Work out the finished part from the listing and answer in its coordinate system (mm). A direction names the side the tool comes from. Coordinates: 2 decimals unless noted, no trailing zeros. Order: outer loops, then holes, each group sorted by start corner. A loop starts at its lowest first (then second) coordinate and runs counter-clockwise, first axis right, second up. Notation, with made-up numbers: M -14,41.5 L -3,41.5 A26 cw -3,57.5 Z; hole C -16.75,-3.75 d3. An arc over 180 degrees is marked long. Use a Markdown table: item, result.
from build123d import *

# Parameters (mm, degrees)
SKETCH_1_R               = 1.65
SKETCH_1_W               = 14
SKETCH_1_H               = 4
SKETCH_1_W_2             = 4
SKETCH_1_H_2             = 10
EXTRUDE_2_DEPTH          = 3
SKETCH_1_3_W             = 34
SKETCH_1_3_H             = 2
SKETCH_1_3_W_2           = 52.77
EXTRUDE_3_DEPTH          = 63
CUT_EXTRUDE_1_DEPTH      = 146.097760148
CUT_EXTRUDE_1_DEPTH_BACK = 146.097760148
SKETCH_2_R               = 2.5
CUT_EXTRUDE_2_DEPTH      = 146.097760148
CUT_EXTRUDE_2_DEPTH_BACK = 146.097760148
SKETCH_4_R               = 2.5


with BuildPart() as part:
    # Sketch 1 → Extrude 2 (new body)
    with BuildSketch(Plane(origin=(0, 0, 0), x_dir=(1, 0, 0), z_dir=(0, 1, 0))):
        Polygon((34, 0), (0, 0), (0, -66.6), (34, -66.6), (57.23, -66.6), (110, -66.6), (110, 0), (57.23, 0), align=None)
        with Locations(Location((11.386101665, -59.551846161, 0), (0, 0, 270))):
            Circle(SKETCH_1_R, mode=Mode.SUBTRACT)
        with Locations(Location((53.38610037, -59.562276184, 0), (0, 0, 270))):
            Circle(SKETCH_1_R, mode=Mode.SUBTRACT)
        with Locations((92.227995582, -61.561806958)):
            Rectangle(SKETCH_1_W, SKETCH_1_H, mode=Mode.SUBTRACT)
        with Locations(Location((85.227995582, -51.6, 0), (0, 0, 270))):
            Circle(SKETCH_1_R, mode=Mode.SUBTRACT)
        with Locations(Location((99.227995582, -51.6, 0), (0, 0, 270))):
            Circle(SKETCH_1_R, mode=Mode.SUBTRACT)
        with Locations(Location((9.892625589, -17.551846161, 0), (0, 0, 270))):
            Circle(SKETCH_1_R, mode=Mode.SUBTRACT)
        with Locations(Location((51.892625589, -17.562276184, 0), (0, 0, 270))):
            Circle(SKETCH_1_R, mode=Mode.SUBTRACT)
        with Locations(Location((85.227995582, -25.6, 0), (0, 0, 270))):
            Circle(SKETCH_1_R, mode=Mode.SUBTRACT)
        with Locations(Location((99.227995582, -25.6, 0), (0, 0, 270))):
            Circle(SKETCH_1_R, mode=Mode.SUBTRACT)
        with Locations((70.219502327, -10)):
            Rectangle(SKETCH_1_W_2, SKETCH_1_H_2, mode=Mode.SUBTRACT)
        with Locations(Location((85, -10, 0), (0, 0, 270))):
            Circle(SKETCH_1_R, mode=Mode.SUBTRACT)
    extrude(amount=EXTRUDE_2_DEPTH)

    # Sketch 1_3 → Extrude 3 (add)
    with BuildSketch(Plane(origin=(0, 0, 0), x_dir=(1, 0, 0), z_dir=(0, 1, 0))):
        with Locations((17, -67.6)):
            Rectangle(SKETCH_1_3_W, SKETCH_1_3_H)
        with Locations((83.615, -67.6)):
            Rectangle(SKETCH_1_3_W_2, SKETCH_1_3_H)
        with Locations((17, 1)):
            Rectangle(SKETCH_1_3_W, SKETCH_1_3_H)
        with Locations((83.615, 1)):
            Rectangle(SKETCH_1_3_W_2, SKETCH_1_3_H)
    extrude(amount=EXTRUDE_3_DEPTH)

    # Sketch 2 → Cut-Extrude 1 (cut, two sides: drawn at the far end of the back side and taken through both)
    with BuildSketch(Plane.XY.offset(68.6).offset(-CUT_EXTRUDE_1_DEPTH_BACK)):
        with Locations((64.73, 32)):
            Circle(SKETCH_2_R)
        with Locations((102.5, 32)):
            Circle(SKETCH_2_R)
        with Locations((64.73, 51.5)):
            Circle(SKETCH_2_R)
        with Locations((102.5, 51.5)):
            Circle(SKETCH_2_R)
        with Locations((26.5, 32)):
            Circle(SKETCH_2_R)
        with Locations((7.5, 32)):
            Circle(SKETCH_2_R)
        with Locations((26.5, 51.5)):
            Circle(SKETCH_2_R)
        with Locations((7.5, 51.5)):
            Circle(SKETCH_2_R)
    extrude(amount=CUT_EXTRUDE_1_DEPTH + CUT_EXTRUDE_1_DEPTH_BACK, mode=Mode.SUBTRACT)

    # Sketch 4 → Cut-Extrude 2 (cut, two sides: drawn at the far end of the back side and taken through both)
    with BuildSketch(Plane(origin=(0, 0, -2), x_dir=(-1, 0, 0), z_dir=(0, 0, -1)).offset(-CUT_EXTRUDE_2_DEPTH_BACK)):
        with Locations((-7.5, 15)):
            Circle(SKETCH_4_R)
    extrude(amount=CUT_EXTRUDE_2_DEPTH + CUT_EXTRUDE_2_DEPTH_BACK, mode=Mode.SUBTRACT)


solid = part.part
1. Flat-ended cylindrical pins translate along their axes: P1, Ø3, axis at x = 26.5, y = 32, coming from the -Z side; P2, Ø5.5, axis at x = 99.23, z = 25.6, coming from the +Y side. Find the tip coordinate at first contact, or state that the pin passes through.
Answers below:
| item | result |
|---|---|
| P1 | through |
| P2 | y = 3 |
2. For faces 1 (the face through (68.22, 1, 10)), 2 (the face through (17, 31, -2)), 3 (the face through (46, 1, 0)), determine the directions among +Z, -Z, +X, -X, +Y, -Y from which every point of the face is accessible in a straight line to the end or side of a thin tool.
Answers below:
| item | result |
|---|---|
| face 1 | +Y, -Y |
| face 2 | -Z, +X, -X, +Y, -Y |
| face 3 | -Z, +Y, -Y |
3. Section B-B on x = 26.5 is taken. Determine the outline of the cut face in (y, z).
Answers below:
| item | result |
|---|---|
| outline | M 0,-2 L 29.5,-2 L 29.5,0 L 3,0 L 3,66.6 L 29.5,66.6 L 29.5,68.6 L 0,68.6 Z; M 34.5,-2 L 49,-2 L 49,0 L 34.5,0 Z; M 34.5,66.6 L 49,66.6 L 49,68.6 L 34.5,68.6 Z; M 54,-2 L 63,-2 L 63,0 L 54,0 Z; M 54,66.6 L 63,66.6 L 63,68.6 L 54,68.6 Z |
4. Section A-A on z = 51.6 is taken. Determine the outline of the cut face in (x, y).
Answers below:
| item | result |
|---|---|
| outline | M 0,0 L 83.58,0 L 83.58,3 L 0,3 Z; M 86.88,0 L 97.58,0 L 97.58,3 L 86.88,3 Z; M 100.88,0 L 110,0 L 110,3 L 100.88,3 Z |
5. Find the intervals of material crossed by probe 1 along X at (y, z) = (51.5, -0.45); probe 2 along Y at (x, z) = (102.5, -0.7); probe 3 along X at (y, z) = (1.95, 25.6), in increasing order.
Answers below:
| item | result |
|---|---|
| probe 1 | 0 to 5, 10 to 24, 29 to 34, 57.23 to 62.23, 67.23 to 100, 105 to 110 |
| probe 2 | 0 to 29.5, 34.5 to 49, 54 to 63 |
| probe 3 | 0 to 83.58, 86.88 to 97.58, 100.88 to 110 |
6. Section C-C on y = 15 is taken. Determine the outline of the cut face in (x, z).
Answers below:
| item | result |
|---|---|
| outline | M 0,-2 L 5,-2 L 5,0 L 0,0 Z; M 0,66.6 L 5,66.6 L 5,68.6 L 0,68.6 Z; M 10,-2 L 34,-2 L 34,0 L 10,0 Z; M 10,66.6 L 34,66.6 L 34,68.6 L 10,68.6 Z; M 57.23,-2 L 110,-2 L 110,0 L 57.23,0 Z; M 57.23,66.6 L 110,66.6 L 110,68.6 L 57.23,68.6 Z |
7. For a pull along Z with two mould halves and no side action, classify faces 4 (the face through (45, 1, 66.6)), 5 (the face through (9.885, 52.251, -1.014)), 6 (the face through (83, 31, -2)), 7 (the face through (83, 33, 0)) as +Z half, -Z half, draft (parallel to the pull), parting line (faces both ways), or undercut.
Answers below:
| item | result |
|---|---|
| face 4 | +Z half |
| face 5 | draft |
| face 6 | -Z half |
| face 7 | undercut |
8. Section D-D on z = 7 is taken. Determine the outline of the cut face in (x, y), then the cut area to 3 significant figures.
Answers below:
| item | result |
|---|---|
| outline | M 0,0 L 68.22,0 L 68.22,3 L 0,3 Z; M 72.22,0 L 110,0 L 110,3 L 72.22,3 Z |
| area | 318 mm² |
